```python
from build123d import *

# Parameters (mm, degrees)
SKETCH_1_R          = 5
EXTRUDE_1_DEPTH     = 4.3
SKETCH_2_R          = 5
SKETCH_2_R_2        = 4
SKETCH_2_R_3        = 2.25
CUT_EXTRUDE_1_DEPTH = 0.3
SKETCH_3_R          = 0.75
EXTRUDE_2_DEPTH     = 0.15
SKETCH_4_R          = 0.5
EXTRUDE_3_DEPTH     = 1.7
FILLET_1_R          = 0.5
FILLET_2_R          = 0.2
FILLET_3_R          = 0.1
SKETCH_5_R          = 5
EXTRUDE_4_DEPTH     = 0.7
EXTRUDE_5_DEPTH     = 3
FILLET_4_R          = 0.1
SKETCH_7_R          = 0.3
EXTRUDE_6_DEPTH     = 3


with BuildPart() as part:
    # Эскиз1 → Бобышка-Вытянуть1 (new body)
    with BuildSketch(Plane(origin=(0, 0, 0), x_dir=(1, 0, 0), z_dir=(0, 1, 0))):
        Circle(SKETCH_1_R)
    extrude(amount=EXTRUDE_1_DEPTH)

    # Эскиз2 → Вырез-Вытянуть1 (cut)
    with BuildSketch(Plane(origin=(0, 4.3, 0), x_dir=(1, 0, 0), z_dir=(0, 1, 0))):
        Circle(SKETCH_2_R)
        Circle(SKETCH_2_R_2, mode=Mode.SUBTRACT)
        Circle(SKETCH_2_R_3)
    extrude(amount=-CUT_EXTRUDE_1_DEPTH, mode=Mode.SUBTRACT)

    # Эскиз3 → Бобышка-Вытянуть2 (add)
    with BuildSketch(Plane(origin=(0, 4, 0), x_dir=(1, 0, 0), z_dir=(0, 1, 0))):
        Circle(SKETCH_3_R)
    extrude(amount=EXTRUDE_2_DEPTH)

    # Эскиз4 → Бобышка-Вытянуть3 (add)
    with BuildSketch(Plane(origin=(0, 4.15, 0), x_dir=(1, 0, 0), z_dir=(0, 1, 0))):
        Circle(SKETCH_4_R)
    extrude(amount=EXTRUDE_3_DEPTH)

    # Скругление1
    fillet_1_edges = [part.edges().sort_by_distance(p)[0] for p in [
        (-0.5, 5.85, 0),
    ]]
    fillet(fillet_1_edges, radius=FILLET_1_R)

    # Скругление2
    fillet_2_edges = [part.edges().sort_by_distance(p)[0] for p in [
        (-5, 0, 0),
        (-5, 4, 0),
    ]]
    fillet(fillet_2_edges, radius=FILLET_2_R)

    # Скругление3
    fillet_3_edges = [part.edges().sort_by_distance(p)[0] for p in [
        (-0.5, 4.15, 0),
    ]]
    fillet(fillet_3_edges, radius=FILLET_3_R)

    # Эскиз5 → Бобышка-Вытянуть4 (add)
    with BuildSketch(Plane.XZ):
        Circle(SKETCH_5_R)
    extrude(amount=EXTRUDE_4_DEPTH)

    # Эскиз6 → Бобышка-Вытянуть5 (add)
    with BuildSketch(Plane.XZ.offset(0.7)):
        with BuildLine():
            Line((0.7, 2.752380788), (0.552112676, 2.170891889))
            ThreePointArc((0.552112676, 2.170891889), (0, 2.24), (-0.552112676, 2.170891889))
            Line((-0.552112676, 2.170891889), (-0.7, 2.752380788))
            ThreePointArc((-0.7, 2.752380788), (0, 2.84), (0.7, 2.752380788))
        make_face()
        with BuildLine():
            Line((0.552112676, -2.170891889), (0.7, -2.752380788))
            ThreePointArc((0.7, -2.752380788), (0, -2.84), (-0.7, -2.752380788))
            Line((-0.7, -2.752380788), (-0.552112676, -2.170891889))
            ThreePointArc((-0.552112676, -2.170891889), (0, -2.24), (0.552112676, -2.170891889))
        make_face()
    extrude(amount=EXTRUDE_5_DEPTH)

    # Скругление4
    fillet_4_edges = [part.edges().sort_by_distance(p)[0] for p in [
        (0.7, -2.2, 2.752380788),
        (-0.7, -2.2, 2.752380788),
        (-0.552112676, -2.2, 2.170891889),
        (0.552112676, -2.2, 2.170891889),
        (-0.7, -2.2, -2.752380788),
        (0.7, -2.2, -2.752380788),
        (0.552112676, -2.2, -2.170891889),
        (-0.552112676, -2.2, -2.170891889),
    ]]
    fillet(fillet_4_edges, radius=FILLET_4_R)

    # Эскиз7 → Бобышка-Вытянуть6 (add)
    with BuildSketch(Plane.XZ.offset(0.7)):
        Circle(SKETCH_7_R)
    extrude(amount=EXTRUDE_6_DEPTH)


solid = part.part
```
Can you work these out from the model? Positions are in its coordinate system, mm. A direction names the side the tool comes from. Give positions to 0.01 mm unless a question says otherwise; leave off trailing zeros. Loops run counter-clockwise (first coordinate to the right, second up) from the corner with the lowest first, then second, coordinate; pieces in that order, holes last. Notation, with made-up numbers: M 72,88 L 113,88 A19 cw 113,112 Z; hole C 4,-21 d9. An arc over 180 degrees is marked long. One line per question, with ' | ' between items. Start each with the question number.
Q1. For faces 1 (the cylindrical face through (0.01, -2.18, 2.24)), 2 (the cylindrical face through (-0.108, 4.792, 0.488)), 3 (the cylindrical face through (-1.08, 1.97, 4.88)), 4 (the cylindrical face through (0.01, -2.18, -2.84)), which set-ups out of +Z, -Z, +X, -X, +Y, -Y let a thin tool reach every point of the face, with its end or its side?
Q2. If we section it at A-A (y = -1): Please give me the cut outline in (x, z).
Q3. If I drill on line 1 (Z direction, x = 0, y = 4.25); line 2 (Z direction, x = 0, y = 4.1), over which ranges is the centre line in solid material (lowest first)? Write a range as from..to.
Q4. For pin 1 Ø2 at (x, z) = (-0.5, -1) entering from +Y; pin 2 Ø1.5 at (y, z) = (2.5, 1) entering from +X; pin 3 Ø2 at (x, z) = (2, -1) entering from +Y, each with a flat end and sliding along its axis, tell me the tip position at first contact or that it passes through.
Q5. If we mould it in two halves opening along X, with no side actions, what happens to faces 5 (the cylindrical face through (-0.29, 4.15, -2.23)), 6 (the cylindrical face through (-0.01, -2.18, 2.84)), 7 (the flat face through (-2, 4, -4))? For each: +X half, -X half, draft (parallel to the pull), parting line (faces both ways), or undercut.
Computed:
1) face 1: -Y | face 2: +Y | face 3: +Y, -Y | face 4: -Z, -Y
2) outline: M -0.67,-2.65 A0.1 ccw -0.6,-2.78 A2.84 ccw 0.6,-2.78 A0.1 ccw 0.67,-2.65 L 0.58,-2.27 A0.1 ccw 0.46,-2.19 A2.24 cw -0.46,-2.19 A0.1 ccw -0.58,-2.27 Z; M -0.67,2.65 L -0.58,2.27 A0.1 ccw -0.46,2.19 A2.24 cw 0.46,2.19 A0.1 ccw 0.58,2.27 L 0.67,2.65 A0.1 ccw 0.6,2.78 A2.84 ccw -0.6,2.78 A0.1 ccw Z; C 0,0 d0.6
3) line 1: z = -4..-2.25, -0.5..0.5, 2.25..4 | line 2: z = -4..-2.25, -0.75..0.75, 2.25..4
4) pin 1: stops at y = 5.84 | pin 2: stops at x = 4.99 | pin 3: stops at y = 4.3
5) face 5: undercut | face 6: parting line | face 7: draft
